Could you check a few things on this drawing? It's one solid part, dimensions in mm from its lowest x, y, z. A direction names the side the tool comes from. Give positions to 0.01 mm unless a question says otherwise; leave off trailing zeros. Loops run counter-clockwise (first coordinate to the right, second up) from the corner with the lowest first, then second, coordinate; pieces in that order, holes last. Notation, with made-up numbers: M 16.5,59.5 L 52.5,59.5 A24 ccw 52.5,69.5 Z; hole C -27.75,18.5 d10. An arc over 180 degrees is marked long. Return JSON: item names as keys, results as strings. Group by question number.
1. If we section it at D-D (z = 15.25): Write out the boundary of the cut face in (x, y), plus the area to 3 significant figures.
2. If we section it at C-C (x = 47.5): Write out the boundary of the cut face in (y, z), plus the area to 3 significant figures.
3. For the marked faces 4 and 5, which set-ups out of +Z, -Z, +X, -X, +Y, -Y let a thin tool reach every point of the face, with its end or its side?
4. If we section it at A-A (z = 8): Write out the boundary of the cut face in (x, y).
5. If we section it at B-B (z = 22): Write out the boundary of the cut face in (x, y), plus the area to 3 significant figures.
6. For pin 1 (6.5 mm diameter, centred on x = 39.58, z = 22, fed in from -Y); pin 2 (9 mm diameter, centred on y = 34, z = 22.5, fed in from -X); pin 3 (2 mm diameter, centred on x = 81.5, y = 33, fed in from -Z), each with a flat end and sliding along its axis, tell me the tip position at first contact or that it passes through.
7. Please list where these lines run through material, in increasing order: line 1 (X direction, y = 51.3, z = 8); line 2 (Y direction, x = 78.5, z = 23.25); line 3 (Y direction, x = 35.5, z = 2.5).
8. If we mould it in two halves opening along Y, with no side actions, what happens to the marked faces 1, 2 and 3? For each: +Y half, -Y half, draft (parallel to the pull), parting line (faces both ways), or undercut.
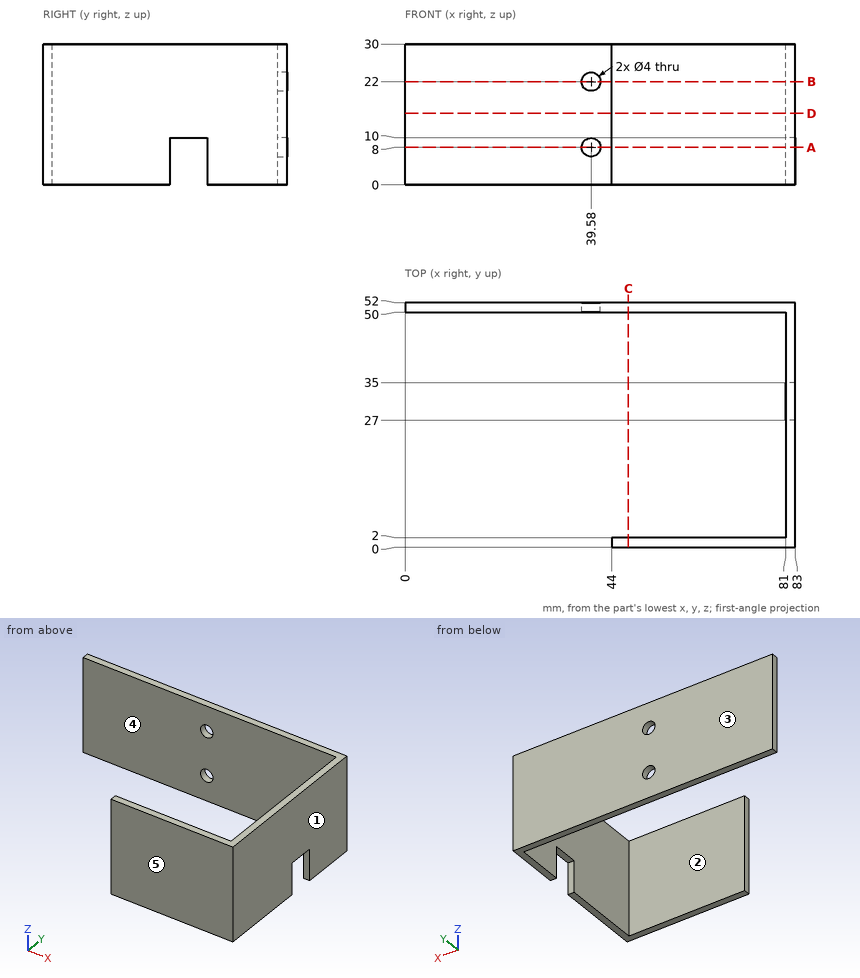
Answer:
{
 "1": {"outline": "M 0,50 L 81,50 L 81,2 L 44,2 L 44,0 L 83,0 L 83,52 L 0,52 Z", "area": "340 mm²"},
 "2": {"outline": "M 0,0 L 2,0 L 2,30 L 0,30 Z; M 50,0 L 52,0 L 52,30 L 50,30 Z", "area": "120 mm²"},
 "3": {"face 4": "+Z, -Z, -X", "face 5": "+Z, -Z, +X, -X, -Y"},
 "4": {"outline": "M 0,50 L 37.58,50 L 37.58,52 L 0,52 Z; M 41.58,50 L 81,50 L 81,35 L 83,35 L 83,52 L 41.58,52 Z; M 44,0 L 83,0 L 83,27 L 81,27 L 81,2 L 44,2 Z"},
 "5": {"outline": "M 0,50 L 37.58,50 L 37.58,52 L 0,52 Z; M 41.58,50 L 81,50 L 81,2 L 44,2 L 44,0 L 83,0 L 83,52 L 41.58,52 Z", "area": "332 mm²"},
 "6": {"pin 1": "stops at y = 50", "pin 2": "stops at x = 81", "pin 3": "stops at z = 10"},
 "7": {"line 1": "x = 0 to 37.58, 41.58 to 83", "line 2": "y = 0 to 2, 50 to 52", "line 3": "y = 50 to 52"},
 "8": {"face 1": "draft", "face 2": "undercut", "face 3": "+Y half"}
}
